For this review, take the finished solid that the model builds, in its own axes (mm). A direction names the side the tool comes from. Give positions to 0.01 mm unless a question says otherwise; leave off trailing zeros. Order: outer loops, then holes, each group sorted by start corner. A loop starts at its lowest first (then second) coordinate and runs counter-clockwise, first axis right, second up.
from build123d import *

# Parameters (mm, degrees)
BOSS_EXTRUDE1_DEPTH = 88.9
SKETCH2_R           = 4
CUT_EXTRUDE1_DEPTH  = 2
SKETCH3_R           = 4
CUT_EXTRUDE2_DEPTH  = 2


with BuildPart() as part:
    # Sketch1 → Boss-Extrude1 (new body)
    with BuildSketch(Plane.XY):
        with BuildLine():
            Line((-40.203883769, 5.937788296), (-44.399042974, 2.127788296))
            ThreePointArc((-44.399042974, 2.127788296), (0, 44.45), (44.399042974, 2.127788296))
            Line((44.399042974, 2.127788296), (40.203883769, 5.937788296))
            ThreePointArc((40.203883769, 5.937788296), (0, 40.64), (-40.203883769, 5.937788296))
        make_face()
    extrude(amount=BOSS_EXTRUDE1_DEPTH)

    # Sketch2 → Cut-Extrude1 (cut)
    with BuildSketch(Plane(origin=(-21.127225221, 23.263011377, 0), x_dir=(0.7402720771062566, 0.6723074087475077, 0), z_dir=(0.6723074087475077, -0.7402720771062566, 0))):
        with Locations((-28.603318705, 66.727309036)):
            Circle(SKETCH2_R)
        with Locations((-28.603318705, 22.172690964)):
            Circle(SKETCH2_R)
    extrude(amount=-CUT_EXTRUDE1_DEPTH, mode=Mode.SUBTRACT)

    # Sketch3 → Cut-Extrude2 (cut)
    with BuildSketch(Plane(origin=(21.127225221, 23.263011377, 0), x_dir=(0.7402720771062566, -0.6723074087475077, 0), z_dir=(-0.6723074087475077, -0.7402720771062566, 0))):
        with Locations((28.603318705, 66.675)):
            Circle(SKETCH3_R)
        with Locations((28.603318705, 22.225)):
            Circle(SKETCH3_R)
    extrude(amount=-CUT_EXTRUDE2_DEPTH, mode=Mode.SUBTRACT)


solid = part.part
1) We need section D-D on y = 36. Give the boundary of the cut face in (x, z), then the cut area to 3 significant figures.
Answer sheet:
outline: (-26.07, 0) - (-18.86, 0) - (-18.86, 88.9) - (-26.07, 88.9) - close; (18.86, 0) - (26.07, 0) - (26.07, 88.9) - (18.86, 88.9) - close
area: 1,280 mm2
2) Draft analysis for pull direction Y (two halves, no side actions). For faces 3 (the face through (3, 41, 88.9)), 4 (the face through (40.15, 7.61, 22.36)), 5 (the face through (42.331, 4.006, 44.178)), state which applies: +Y half, -Y half, draft (parallel to the pull), parting line (faces both ways), or undercut.
Answer sheet:
face 3: draft
face 4: undercut
face 5: -Y half
3) We need section C-C on x = 0. Give the boundary of the cut face in (y, z).
Answer sheet:
outline: (40.64, 0) - (44.45, 0) - (44.45, 88.9) - (40.64, 88.9) - close
4) We need section A-A on y = 14. Give the boundary of the cut face in (x, z), then the cut area to 3 significant figures.
Answer sheet:
outline: (-42.19, 0) - (-38.15, 0) - (-38.15, 88.9) - (-42.19, 88.9) - close; (38.15, 0) - (42.19, 0) - (42.19, 88.9) - (38.15, 88.9) - close
area: 717 mm2
5) To check wall thickness, follow line 1 (X direction, y = 22, z = 39); line 2 (X direction, y = 11.5, z = 78); line 3 (Y direction, x = 0.5, z = 46). State the ranges of each line that lie inside material, in increasing order.
Answer sheet:
line 1: x = -38.62 to -34.17, 34.17 to 38.62
line 2: x = -42.94 to -38.98, 38.98 to 42.94
line 3: y = 40.64 to 44.45
6) Tool access review of faces 1 (the face through (-42.27, 4.06, 44.18)), 2 (the face through (-0.95, 44.44, 43.83)): name each direction out of +Z, -Z, +X, -X, +Y, -Y from which nothing blocks a thin tool from reaching the whole face with its end or side.
Answer sheet:
face 1: +Z, -Z, -Y
face 2: +Z, -Z, +Y
7) We need section B-B on z = 66. Give the boundary of the cut face in (x, y).
Answer sheet:
outline: (-44.16, 5.04) - (-40.73, 8.16) - (-39.98, 7.32) arc R40.64 cw to (39.97, 7.33) - (40.73, 8.16) - (44.16, 5.04) arc R44.45 ccw to start
8) Clearance check with flat-ended pins moving along their axes: pin 1 (4 mm diameter, centred on x = 28, z = 61.5, fed in from -Y); pin 2 (3 mm diameter, centred on x = -21, z = 49, fed in from -Y); pin 3 (12 mm diameter, centred on x = -6.5, z = 25, fed in from -Y); pin 4 (4 mm diameter, centred on x = -26.5, y = 38.5, fed in from -Z). State where each tip first meets the part, or that it passes through.
Answer sheet:
pin 1: stops at y = 27.42
pin 2: stops at y = 33.84
pin 3: stops at y = 38.67
pin 4: passes through
